```python
from build123d import *

# Parameters (mm, degrees)
F0_R     = 63.5
F0_R_2   = 19.05
F1_DEPTH = 12.7
F3_D     = 17.78


# Not quite as in the source:
# - a fillet or chamfer that OpenCascade refuses, or shapes differently, is made with other operations: its cross-section is extruded or revolved along the edge and cut away or added


with BuildPart() as f1:
    # F0 (on Top) → F1 (new body)
    with BuildSketch(Plane.XY):
        Circle(F0_R)
        Circle(F0_R_2, mode=Mode.SUBTRACT)
    extrude(amount=F1_DEPTH)

    # F3 (through all)
    with Locations(Plane(origin=(0, 0, 0), x_dir=(1, 0, 0), z_dir=(0, 0, -1))):
        with Locations((0, -38.1), (-38.1, 0), (0, 38.1), (38.1, 0)):
            Hole(F3_D / 2)

    # F4: chamfer of 6.35 on 12 edges, made by hand

    # F4_s1 → F4_t2 (revolve, cut)
    with BuildSketch(Plane.XZ):
        Polygon((25.4, 0), (19.05, 6.35), (19.05, 0), align=None)
    revolve(axis=Axis((0, 0, 0), (0, 0, 1)), mode=Mode.SUBTRACT)

    # F4_s3 → F4_t4 (revolve, cut)
    with BuildSketch(Plane.XZ):
        Polygon((25.4, 12.7), (19.05, 6.35), (19.05, 12.7), align=None)
    revolve(axis=Axis((0, 0, 12.7), (0, 0, 1)), mode=Mode.SUBTRACT)

    # F4_s5 → F4_t6 (revolve, cut)
    with BuildSketch(Plane.XZ):
        Polygon((63.5, 6.35), (57.15, 12.7), (63.5, 12.7), align=None)
    revolve(axis=Axis((0, 0, 12.7), (0, 0, 1)), mode=Mode.SUBTRACT)

    # F4_s7 → F4_t8 (revolve, cut)
    with BuildSketch(Plane.XZ):
        Polygon((63.5, 6.35), (57.15, 0), (63.5, 0), align=None)
    revolve(axis=Axis((0, 0, 0), (0, 0, 1)), mode=Mode.SUBTRACT)

    # F4_s9 → F4_t10 (revolve, cut)
    with BuildSketch(Plane.XZ.offset(38.1)):
        Polygon((15.24, 0), (8.89, 6.35), (8.89, 0), align=None)
    revolve(axis=Axis((0, -38.1, 0), (0, 0, -1)), mode=Mode.SUBTRACT)

    # F4_s11 → F4_t12 (revolve, cut)
    with BuildSketch(Plane.XZ):
        Polygon((-22.86, 0), (-29.21, 6.35), (-29.21, 0), align=None)
    revolve(axis=Axis((-38.1, 0, 0), (0, 0, -1)), mode=Mode.SUBTRACT)

    # F4_s13 → F4_t14 (revolve, cut)
    with BuildSketch(Plane.XZ):
        Polygon((53.34, 0), (46.99, 6.35), (46.99, 0), align=None)
    revolve(axis=Axis((38.1, 0, 0), (0, 0, -1)), mode=Mode.SUBTRACT)

    # F4_s15 → F4_t16 (revolve, cut)
    with BuildSketch(Plane.XZ.offset(-38.1)):
        Polygon((15.24, 0), (8.89, 6.35), (8.89, 0), align=None)
    revolve(axis=Axis((0, 38.1, 0), (0, 0, -1)), mode=Mode.SUBTRACT)

    # F4_s17 → F4_t18 (revolve, cut)
    with BuildSketch(Plane.XZ.offset(38.1)):
        Polygon((15.24, 12.7), (8.89, 6.35), (8.89, 12.7), align=None)
    revolve(axis=Axis((0, -38.1, 12.7), (0, 0, -1)), mode=Mode.SUBTRACT)

    # F4_s19 → F4_t20 (revolve, cut)
    with BuildSketch(Plane.XZ):
        Polygon((-22.86, 12.7), (-29.21, 6.35), (-29.21, 12.7), align=None)
    revolve(axis=Axis((-38.1, 0, 12.7), (0, 0, -1)), mode=Mode.SUBTRACT)

    # F4_s21 → F4_t22 (revolve, cut)
    with BuildSketch(Plane.XZ):
        Polygon((53.34, 12.7), (46.99, 6.35), (46.99, 12.7), align=None)
    revolve(axis=Axis((38.1, 0, 12.7), (0, 0, -1)), mode=Mode.SUBTRACT)

    # F4_s23 → F4_t24 (revolve, cut)
    with BuildSketch(Plane.XZ.offset(-38.1)):
        Polygon((15.24, 12.7), (8.89, 6.35), (8.89, 12.7), align=None)
    revolve(axis=Axis((0, 38.1, 12.7), (0, 0, -1)), mode=Mode.SUBTRACT)


solid = f1.part
```
Source: CAD feature listing. Evaluate the final solid. Frame: model axes, mm. Give positions to 0.01 mm unless a question says otherwise; leave off trailing zeros. Loops run counter-clockwise (first coordinate to the right, second up) from the corner with the lowest first, then second, coordinate; pieces in that order, holes last. Notation, with made-up numbers: (28, -26.75) -> (69, -26.75) arc R30 cw to (69, 9.25) -> close; hole circle Ø1 at (79.5, 68.25). An arc over 180 degrees is marked (long way). Use a Markdown table: item, result. Add a question column.
(1) Pull-direction query (X, two-part tool) for faces 1 (the face through (-1.2, -47.22, 6.66)), 2 (the face through (25, -12, 0)), 3 (the face through (-12.46, -56.09, 0.31)); classes: +X half, -X half, draft (parallel to the pull), parting line (faces both ways), or undercut.
(2) Section query B-B (z = 9). Output: boundary loops of the cut face in (x, y).
(3) Section query A-A (x = 0). Output: boundary loops of the cut face in (y, z).
(4) Ray query, line 1 (X direction, y = -3.5, z = 10.75); line 2 (Y direction, x = 0.5, z = 4.5); line 3 (X direction, y = -1.5, z = 1.5). Return the intervals inside material, ascending.
(5) First-contact query: pin 1 Ø2 at (x, y) = (-26, -10.5) entering from -Z; pin 2 Ø5 at (y, z) = (17.5, 8.5) entering from +X; pin 3 Ø1 at (y, z) = (-10, 6) entering from -X; pin 4 Ø3 at (x, z) = (-20.5, 1.5) entering from -Y. Flat tips, straight axial feed; report the tip coordinate or a pass-through.
Checked values:
| question | item | result |
|---|---|---|
| 1 | face 1 | undercut |
| 1 | face 2 | draft |
| 1 | face 3 | parting line |
| 2 | outline | circle Ø121.7 at (0, 0); hole circle Ø23.08 at (-38.1, 0); hole circle Ø43.4 at (0, 0); hole circle Ø23.08 at (0, -38.1); hole circle Ø23.08 at (0, 38.1); hole circle Ø23.08 at (38.1, 0) |
| 3 | outline | (-63.5, 6.35) -> (-57.15, 0) -> (-53.34, 0) -> (-46.99, 6.35) -> (-53.34, 12.7) -> (-57.15, 12.7) -> close; (-29.21, 6.35) -> (-24.13, 1.27) -> (-19.05, 6.35) -> (-24.13, 11.43) -> close; (19.05, 6.35) -> (24.13, 1.27) -> (29.21, 6.35) -> (24.13, 11.43) -> close; (46.99, 6.35) -> (53.34, 0) -> (57.15, 0) -> (63.5, 6.35) -> (57.15, 12.7) -> (53.34, 12.7) -> close |
| 4 | line 1 | -59 to -50.92, -25.28 to -23.19, 23.19 to 25.28, 50.92 to 59 |
| 4 | line 2 | -61.65 to -48.83, -27.37 to -20.89, 20.89 to 27.37, 48.83 to 61.65 |
| 4 | line 3 | -58.63 to -51.76, -24.44 to -23.85, 23.85 to 24.44, 51.76 to 58.63 |
| 5 | pin 1 | z = 0 |
| 5 | pin 2 | x = 61.39 |
| 5 | pin 3 | x = -62.76 |
| 5 | pin 4 | y = -56.64 |
